Verification items for the finished model (mm, model axes). Face numbers are marked on the shaded views. A direction names the side the tool comes from. Coordinates: 2 decimals unless noted, no trailing zeros. Order: outer loops, then holes, each group sorted by start corner. A loop starts at its lowest first (then second) coordinate and runs counter-clockwise, first axis right, second up. Notation, with made-up numbers: M -32,1.25 L -14,1.25 A22 cw -14,23.25 Z; hole C -10.75,14.25 d4. An arc over 180 degrees is marked long. Answer as a JSON object with one key per item and string values. Group by question number.
(1) Cross-section at B-B (y = 10). Enter the section's corners in (x, z).
(2) Gauge pin test, flat ends, axial feed: pin 1 Ø6 at (x, y) = (-6.5, 1.5) entering from +Z; pin 2 Ø1.5 at (x, z) = (-2.5, -134) entering from -Y; pin 3 Ø3.5 at (x, z) = (-0.5, -150) entering from -Y. Record the tip position at first contact, or that the pin passes through.
(3) Cross-section at A-A (x = 0). Enter the section's corners in (y, z), plus the area to 3 significant figures.
(4) Mould release check, pull along X, two halves, no side actions. Record for the marked faces 1, 2, 3 and 4: released by +X, released by -X, zero draft, split by the parting line, or undercut.
(5) Cross-section at C-C (y = -1). Enter the section's corners in (x, z), plus the area to 3 significant figures.
(6) Access from +Z, -Z, +X, -X, +Y, -Y to the whole of each face (thin tool, end or side, straight path). Record for the marked faces 5 and 6.
(7) Cross-section at D-D (z = -148.5). Count the separate pieces of the cut face and the enclosed holes in it, plus the area to 3 significant figures.
(8) Material ranges on line 1 (Y direction, x = 6.75, z = -144); line 2 (Y direction, x = 0, z = -159); line 3 (Y direction, x = -4.25, z = -167.5), recorded low to high.
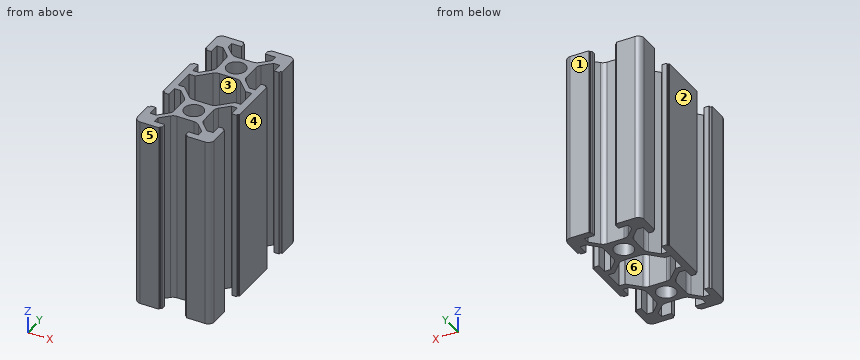
from build123d import *

# Parameters (mm, degrees)
CROQUIS3_R              = 2.5
SALIENTE_EXTRUIR3_DEPTH = 175
SKETCH1_W               = 4.862742591
SKETCH1_H               = 300
SKETCH1_W_2             = 1.5
SKETCH1_W_3             = 0.035786438
CUT_EXTRUDE3_DEPTH      = 100


with BuildPart() as part:
    # Croquis3 → Saliente-Extruir3 (new, symmetric)
    with BuildSketch(Plane.XY):
        with BuildLine():
            Line((-9.5, -13.101470971), (-9.5, -13.401470971))
            ThreePointArc((-9.5, -13.401470971), (-9.558578644, -13.542892327), (-9.7, -13.601470971))
            Line((-9.7, -13.601470971), (-10, -13.601470971))
            Line((-10, -13.601470971), (-10, -18.5))
            ThreePointArc((-10, -18.5), (-9.560660172, -19.560660172), (-8.5, -20))
            Line((-8.5, -20), (-3.601470971, -20))
            Line((-3.601470971, -20), (-3.601470971, -19.7))
            ThreePointArc((-3.601470971, -19.7), (-3.542892327, -19.558578644), (-3.401470971, -19.5))
            Line((-3.401470971, -19.5), (-3.101470971, -19.5))
            Line((-3.101470971, -19.5), (-3.101470971, -18.2))
            Line((-3.101470971, -18.2), (-5.751470971, -18.2))
            Line((-5.751470971, -18.2), (-5.751470971, -16.6))
            Line((-5.751470971, -16.6), (-3.637257409, -14.485786438))
            ThreePointArc((-3.637257409, -14.485786438), (-2.988410711, -14.052240935), (-2.223043846, -13.9))
            Line((-2.223043846, -13.9), (2.223043846, -13.9))
            ThreePointArc((2.223043846, -13.9), (2.988410711, -14.052240935), (3.637257409, -14.485786438))
            Line((3.637257409, -14.485786438), (5.751470971, -16.6))
            Line((5.751470971, -16.6), (5.751470971, -18.2))
            Line((5.751470971, -18.2), (3.101470971, -18.2))
            Line((3.101470971, -18.2), (3.101470971, -19.5))
            Line((3.101470971, -19.5), (3.401470971, -19.5))
            ThreePointArc((3.401470971, -19.5), (3.542892327, -19.558578644), (3.601470971, -19.7))
            Line((3.601470971, -19.7), (3.601470971, -20))
            Line((3.601470971, -20), (8.5, -20))
            ThreePointArc((8.5, -20), (9.560660172, -19.560660172), (10, -18.5))
            Line((10, -18.5), (10, -13.601470971))
            Line((10, -13.601470971), (9.7, -13.601470971))
            ThreePointArc((9.7, -13.601470971), (9.558578644, -13.542892327), (9.5, -13.401470971))
            Line((9.5, -13.401470971), (9.5, -13.101470971))
            Line((9.5, -13.101470971), (8.2, -13.101470971))
            Line((8.2, -13.101470971), (8.2, -15.751470971))
            Line((8.2, -15.751470971), (6.6, -15.751470971))
            Line((6.6, -15.751470971), (4.485786438, -13.637257409))
            ThreePointArc((4.485786438, -13.637257409), (4.052240935, -12.988410711), (3.9, -12.223043846))
            Line((3.9, -12.223043846), (3.9, -7.776956154))
            ThreePointArc((3.9, -7.776956154), (4.052507548, -7.010945946), (4.486771639, -6.361758076))
            Line((4.486771639, -6.361758076), (6.6, -4.251470971))
            Line((6.6, -4.251470971), (8.2, -4.251470971))
            Line((8.2, -4.251470971), (8.2, -6.901470971))
            Line((8.2, -6.901470971), (9.5, -6.901470971))
            Line((9.5, -6.901470971), (9.5, -6.601470971))
            ThreePointArc((9.5, -6.601470971), (9.558578644, -6.460049615), (9.7, -6.401470971))
            Line((9.7, -6.401470971), (10, -6.401470971))
            Line((10, -6.401470971), (10, 6.401470971))
            Line((10, 6.401470971), (9.7, 6.401470971))
            ThreePointArc((9.7, 6.401470971), (9.558578644, 6.460049615), (9.5, 6.601470971))
            Line((9.5, 6.601470971), (9.5, 6.901470971))
            Line((9.5, 6.901470971), (8.2, 6.901470971))
            Line((8.2, 6.901470971), (8.2, 4.251470971))
            Line((8.2, 4.251470971), (6.6, 4.251470971))
            Line((6.6, 4.251470971), (4.486771639, 6.361758076))
            ThreePointArc((4.486771639, 6.361758076), (4.052507548, 7.010945946), (3.9, 7.776956154))
            Line((3.9, 7.776956154), (3.9, 12.223043846))
            ThreePointArc((3.9, 12.223043846), (4.052240935, 12.988410711), (4.485786438, 13.637257409))
            Line((4.485786438, 13.637257409), (6.6, 15.751470971))
            Line((6.6, 15.751470971), (8.2, 15.751470971))
            Line((8.2, 15.751470971), (8.2, 13.101470971))
            Line((8.2, 13.101470971), (9.5, 13.101470971))
            Line((9.5, 13.101470971), (9.5, 13.401470971))
            ThreePointArc((9.5, 13.401470971), (9.558578644, 13.542892327), (9.7, 13.601470971))
            Line((9.7, 13.601470971), (10, 13.601470971))
            Line((10, 13.601470971), (10, 18.5))
            ThreePointArc((10, 18.5), (9.560660172, 19.560660172), (8.5, 20))
            Line((8.5, 20), (3.601470971, 20))
            Line((3.601470971, 20), (3.601470971, 19.7))
            ThreePointArc((3.601470971, 19.7), (3.542892327, 19.558578644), (3.401470971, 19.5))
            Line((3.401470971, 19.5), (3.101470971, 19.5))
            Line((3.101470971, 19.5), (3.101470971, 18.2))
            Line((3.101470971, 18.2), (5.751470971, 18.2))
            Line((5.751470971, 18.2), (5.751470971, 16.6))
            Line((5.751470971, 16.6), (3.637257409, 14.485786438))
            ThreePointArc((3.637257409, 14.485786438), (2.988410711, 14.052240935), (2.223043846, 13.9))
            Line((2.223043846, 13.9), (-2.223043846, 13.9))
            ThreePointArc((-2.223043846, 13.9), (-2.988410711, 14.052240935), (-3.637257409, 14.485786438))
            Line((-3.637257409, 14.485786438), (-5.751470971, 16.6))
            Line((-5.751470971, 16.6), (-5.751470971, 18.2))
            Line((-5.751470971, 18.2), (-3.101470971, 18.2))
            Line((-3.101470971, 18.2), (-3.101470971, 19.5))
            Line((-3.101470971, 19.5), (-3.401470971, 19.5))
            ThreePointArc((-3.401470971, 19.5), (-3.542892327, 19.558578644), (-3.601470971, 19.7))
            Line((-3.601470971, 19.7), (-3.601470971, 20))
            Line((-3.601470971, 20), (-8.5, 20))
            ThreePointArc((-8.5, 20), (-9.560660172, 19.560660172), (-10, 18.5))
            Line((-10, 18.5), (-10, 13.601470971))
            Line((-10, 13.601470971), (-9.7, 13.601470971))
            ThreePointArc((-9.7, 13.601470971), (-9.558578644, 13.542892327), (-9.5, 13.401470971))
            Line((-9.5, 13.401470971), (-9.5, 13.101470971))
            Line((-9.5, 13.101470971), (-8.2, 13.101470971))
            Line((-8.2, 13.101470971), (-8.2, 15.751470971))
            Line((-8.2, 15.751470971), (-6.6, 15.751470971))
            Line((-6.6, 15.751470971), (-4.485786438, 13.637257409))
            ThreePointArc((-4.485786438, 13.637257409), (-4.052240935, 12.988410711), (-3.9, 12.223043846))
            Line((-3.9, 12.223043846), (-3.9, 7.776956154))
            ThreePointArc((-3.9, 7.776956154), (-4.052507548, 7.010945946), (-4.486771639, 6.361758076))
            Line((-4.486771639, 6.361758076), (-6.6, 4.251470971))
            Line((-6.6, 4.251470971), (-8.2, 4.251470971))
            Line((-8.2, 4.251470971), (-8.2, 6.901470971))
            Line((-8.2, 6.901470971), (-9.5, 6.901470971))
            Line((-9.5, 6.901470971), (-9.5, 6.601470971))
            ThreePointArc((-9.5, 6.601470971), (-9.558578644, 6.460049615), (-9.7, 6.401470971))
            Line((-9.7, 6.401470971), (-10, 6.401470971))
            Line((-10, 6.401470971), (-10, -6.401470971))
            Line((-10, -6.401470971), (-9.7, -6.401470971))
            ThreePointArc((-9.7, -6.401470971), (-9.558578644, -6.460049615), (-9.5, -6.601470971))
            Line((-9.5, -6.601470971), (-9.5, -6.901470971))
            Line((-9.5, -6.901470971), (-8.2, -6.901470971))
            Line((-8.2, -6.901470971), (-8.2, -4.251470971))
            Line((-8.2, -4.251470971), (-6.6, -4.251470971))
            Line((-6.6, -4.251470971), (-4.486771639, -6.361758076))
            ThreePointArc((-4.486771639, -6.361758076), (-4.052507548, -7.010945946), (-3.9, -7.776956154))
            Line((-3.9, -7.776956154), (-3.9, -12.223043846))
            ThreePointArc((-3.9, -12.223043846), (-4.052240935, -12.988410711), (-4.485786438, -13.637257409))
            Line((-4.485786438, -13.637257409), (-6.6, -15.751470971))
            Line((-6.6, -15.751470971), (-8.2, -15.751470971))
            Line((-8.2, -15.751470971), (-8.2, -13.101470971))
            Line((-8.2, -13.101470971), (-9.5, -13.101470971))
        make_face()
        with Locations((0, -10)):
            Circle(CROQUIS3_R, mode=Mode.SUBTRACT)
        with Locations(Location((0, 10, 0), (0, 0, 180))):
            Circle(CROQUIS3_R, mode=Mode.SUBTRACT)
        with BuildLine():
            Line((-3.636272208, -5.515198077), (-6.6, -2.555595292))
            Line((-6.6, -2.555595292), (-8.2, -2.555595292))
            Line((-8.2, -2.555595292), (-8.2, 2.555595292))
            Line((-8.2, 2.555595292), (-6.6, 2.555595292))
            Line((-6.6, 2.555595292), (-3.636272208, 5.515198077))
            ThreePointArc((-3.636272208, 5.515198077), (-2.987767275, 5.948025454), (-2.223043846, 6.1))
            Line((-2.223043846, 6.1), (2.223043846, 6.1))
            ThreePointArc((2.223043846, 6.1), (2.987767275, 5.948025454), (3.636272208, 5.515198077))
            Line((3.636272208, 5.515198077), (6.6, 2.555595292))
            Line((6.6, 2.555595292), (8.2, 2.555595292))
            Line((8.2, 2.555595292), (8.2, -2.555595292))
            Line((8.2, -2.555595292), (6.6, -2.555595292))
            Line((6.6, -2.555595292), (3.636272208, -5.515198077))
            ThreePointArc((3.636272208, -5.515198077), (2.987767275, -5.948025454), (2.223043846, -6.1))
            Line((2.223043846, -6.1), (-2.223043846, -6.1))
            ThreePointArc((-2.223043846, -6.1), (-2.987767275, -5.948025454), (-3.636272208, -5.515198077))
        make_face(mode=Mode.SUBTRACT)
    extrude(amount=SALIENTE_EXTRUIR3_DEPTH, both=True)

    # Sketch1 → Cut-Extrude3 (cut)
    with BuildSketch(Plane(origin=(0, 20, 0), x_dir=(1, 0, 0), z_dir=(0, 1, 0))):
        Polygon((3.637257409, -175), (8.5, -175), (10, -175), (10, 125), (3.637257409, 125), align=None)
        Polygon((2.223043846, -175), (3.601470971, -175), (3.601470971, 125), (-3.601470971, 125), (-3.601470971, -175), (-2.223043846, -175), align=None)
        with Locations((-6.068628705, -25)):
            Rectangle(SKETCH1_W, SKETCH1_H)
        with Locations((-9.25, -25)):
            Rectangle(SKETCH1_W_2, SKETCH1_H)
        with Locations((-3.61936419, -25)):
            Rectangle(SKETCH1_W_3, SKETCH1_H)
        with Locations((3.61936419, -25)):
            Rectangle(SKETCH1_W_3, SKETCH1_H)
    extrude(amount=-CUT_EXTRUDE3_DEPTH, mode=Mode.SUBTRACT)


solid = part.part
Taken from the geometry:
{
 "1": {"outline": "M -3.9,-175 L -2.5,-175 L -2.5,-125 L -3.9,-125 Z; M 2.5,-175 L 3.9,-175 L 3.9,-125 L 2.5,-125 Z"},
 "2": {"pin 1": "stops at z = -125", "pin 2": "stops at y = -19.5", "pin 3": "stops at y = -13.9"},
 "3": {"outline": "M -13.9,-175 L -12.5,-175 L -12.5,-125 L -13.9,-125 Z; M -7.5,-175 L -6.1,-175 L -6.1,-125 L -7.5,-125 Z; M 6.1,-175 L 7.5,-175 L 7.5,-125 L 6.1,-125 Z; M 12.5,-175 L 13.9,-175 L 13.9,-125 L 12.5,-125 Z", "area": "280 mm²"},
 "4": {"face 1": "zero draft", "face 2": "released by -X", "face 3": "undercut", "face 4": "released by +X"},
 "5": {"outline": "M -10,-175 L -8.2,-175 L -8.2,-125 L -10,-125 Z; M 8.2,-175 L 10,-175 L 10,-125 L 8.2,-125 Z", "area": "180 mm²"},
 "6": {"face 5": "+Z, -Z, +X, -X, -Y", "face 6": "+Z, -Z"},
 "7": {"separate pieces": "1", "enclosed holes": "3", "area": "285 mm²"},
 "8": {"line 1": "y = -20 to -15.75, -4.25 to -2.56, 2.56 to 4.25, 15.75 to 20", "line 2": "y = -13.9 to -12.5, -7.5 to -6.1, 6.1 to 7.5, 12.5 to 13.9", "line 3": "y = -20 to -18.2, -15.1 to -13.35, -6.65 to -4.9, 4.9 to 6.65, 13.35 to 15.1, 18.2 to 20"}
}
